Geometry check sheet. Reference: the model listing, model coordinates, mm. A direction names the side the tool comes from. Round coordinates to 2 decimals unless told otherwise and drop trailing zeros. Order: outer loops, then holes, each group sorted by start corner. A loop starts at its lowest first (then second) coordinate and runs counter-clockwise, first axis right, second up. Notation, with made-up numbers: M 16.5,65 L 26.5,65 A29 ccw 26.5,87 Z; hole C 65.5,-23 d5. An arc over 180 degrees is marked long. Answer as a JSON object with one key per item and string values. Group by question number.
```python
from build123d import *

# Parameters (mm, degrees)
SKETCH1_W           = 130
SKETCH1_H           = 130
BOSS_EXTRUDE1_DEPTH = 15
SKETCH2_W           = 15
SKETCH2_H           = 130
BOSS_EXTRUDE2_DEPTH = 5
CUT_EXTRUDE2_DEPTH  = 5
CUT_EXTRUDE3_DEPTH  = 120.725284495
SKETCH8_W           = 27
SKETCH8_H           = 85
CUT_EXTRUDE5_DEPTH  = 10


with BuildPart() as part:
    # Sketch1 → Boss-Extrude1 (new body)
    with BuildSketch(Plane.XY):
        with Locations((-9.518828452, -13.870292887)):
            Rectangle(SKETCH1_W, SKETCH1_H)
    extrude(amount=BOSS_EXTRUDE1_DEPTH)

    # Sketch2 → Boss-Extrude2 (add)
    with BuildSketch(Plane.XY.offset(15)):
        with Locations((62.981171548, -13.870292887)):
            Rectangle(SKETCH2_W, SKETCH2_H)
        with Locations((-82.018828452, -13.870292887)):
            Rectangle(SKETCH2_W, SKETCH2_H)
    extrude(amount=-BOSS_EXTRUDE2_DEPTH)

    # Sketch3 → Cut-Extrude2 (cut)
    with BuildSketch(Plane.XY.offset(15)):
        Polygon((-9.518828452, -13.870292887), (-59.518828452, 26.754707113), (-59.518828452, -54.495292887), align=None)
        Polygon((-59.518828452, 36.129707113), (-59.518828452, 26.754707113), (-9.518828452, -13.870292887), (40.481171548, 26.754707113), (40.481171548, 36.129707113), align=None)
        Polygon((40.481171548, -54.495292887), (-9.518828452, -13.870292887), (-59.518828452, -54.495292887), (-59.518828452, -63.870292887), (40.481171548, -63.870292887), align=None)
        Polygon((40.481171548, 26.754707113), (-9.518828452, -13.870292887), (40.481171548, -54.495292887), align=None)
    extrude(amount=-CUT_EXTRUDE2_DEPTH, mode=Mode.SUBTRACT)

    # Sketch5 → Cut-Extrude3 (cut, through all)
    with BuildSketch(Plane.XY.offset(10)):
        Polygon((-47.518828452, 24.129707113), (-47.518828452, -51.870292887), (-9.518828452, -13.870292887), align=None)
        Polygon((-47.518828452, 24.129707113), (-9.518828452, -13.870292887), (28.481171548, 24.129707113), (28.481171548, 28.629707113), (-47.518828452, 28.629707113), align=None)
        Polygon((28.481171548, 24.129707113), (-9.518828452, -13.870292887), (28.481171548, -51.870292887), align=None)
        Polygon((-9.518828452, -13.870292887), (-47.518828452, -51.870292887), (-47.518828452, -56.370292887), (28.481171548, -56.370292887), (28.481171548, -51.870292887), align=None)
    extrude(amount=-CUT_EXTRUDE3_DEPTH, mode=Mode.SUBTRACT)

    # Sketch8 → Cut-Extrude5 (cut)
    with BuildSketch(Plane(origin=(0, 0, 0), x_dir=(-1, 0, 0), z_dir=(0, 0, -1))):
        with Locations((61.018828452, -13.870292887)):
            Rectangle(SKETCH8_W, SKETCH8_H)
        with Locations((-41.981171548, -13.870292887)):
            Rectangle(SKETCH8_W, SKETCH8_H)
    extrude(amount=-CUT_EXTRUDE5_DEPTH, mode=Mode.SUBTRACT)


solid = part.part
```
1) Thickness scan on line 1 along Y through (x, z) = (-11, 1); line 2 along Y through (x, z) = (-36, 12.5); line 3 along X through (y, z) = (15, 11). Record the ranges inside material, lowest first. Write a range as [from, to].
2) Sectioned sample at A-A (x = 7). Record the boundary of the cut face in (y, z).
3) Sectioned sample at B-B (z = 4). Record the boundary of the cut face in (x, y).
4) Sectioned sample at C-C (y = -32). Record the boundary of the cut face in (x, z), then the cut area to 3 significant figures.
5) Release check for a two-part mould opening along Y. For faces 1 (the flat face through (-89.519, -15, 13)), 2 (the flat face through (-9, 28.63, 5)), 3 (the flat face through (-11, -78.87, 8)) record: +Y half, -Y half, draft (parallel to the pull), parting line (faces both ways), or undercut.
6) Set-up check for faces 4 (the flat face through (55.481, -68, 5)), 5 (the flat face through (-64, -13, 15)), 6 (the flat face through (-74.519, 40, 5)), 7 (the flat face through (-11, 51.13, 8)), 8 (the flat face through (40.481, -15, 13)): record each of +Z, -Z, +X, -X, +Y, -Y from which the full face is reachable in a straight line by a thin tool's end or side.
7) Sectioned sample at D-D (y = 31.5). Record the boundary of the cut face in (x, z).
8) Go/stop test with flat-tipped pins: P1, Ø6, axis at x = 27, y = -56.5, coming from the +Z side; P2, Ø5, axis at y = -66.5, z = 5, coming from the -X side; P3, Ø5, axis at y = 35, z = 5, coming from the +X side. Record where each tip stops, or that it passes through.
Final values:
{
 "1": {"line 1": "y = [-78.87, -56.37], [28.63, 51.13]", "line 2": "y = [-78.87, -63.87], [36.13, 51.13]", "line 3": "x = [-89.52, -59.52], [40.48, 70.48]"},
 "2": {"outline": "M -78.87,0 L -56.37,0 L -56.37,10 L -63.87,10 L -63.87,15 L -78.87,15 Z; M 28.63,0 L 51.13,0 L 51.13,15 L 36.13,15 L 36.13,10 L 28.63,10 Z"},
 "3": {"outline": "M -74.52,-78.87 L 55.48,-78.87 L 55.48,-56.37 L -74.52,-56.37 Z; M -74.52,28.63 L 55.48,28.63 L 55.48,51.13 L -74.52,51.13 Z"},
 "4": {"outline": "M -89.52,10 L -59.52,10 L -59.52,15 L -89.52,15 Z; M 40.48,10 L 70.48,10 L 70.48,15 L 40.48,15 Z", "area": "300 mm^2"},
 "5": {"face 1": "draft", "face 2": "undercut", "face 3": "-Y half"},
 "6": {"face 4": "-Z, +X, +Y, -Y", "face 5": "+Z, +X, -X, +Y, -Y", "face 6": "-Z, -X, +Y, -Y", "face 7": "+Z, -Z, +X, -X, +Y", "face 8": "+Z"},
 "7": {"outline": "M -89.52,10 L -74.52,10 L -74.52,0 L 55.48,0 L 55.48,10 L 70.48,10 L 70.48,15 L 40.48,15 L 40.48,10 L -59.52,10 L -59.52,15 L -89.52,15 Z"},
 "8": {"P1": "stops at z = 10", "P2": "stops at x = -74.52", "P3": "stops at x = 55.48"}
}
